Autodesk Inventor part; units mm, degrees
ref_plane "Work Plane2" through (0, 12.5, 0) normal (0, 1, 0) x (1, 0, 0)
ref_plane "YZ Plane" through (0, 0, 0) normal (1, 0, 0) x (0, 1, 0)
ref_plane "XZ Plane" through (0, 0, 0) normal (0, 1, 0) x (-1, 0, 0)
sketch "Sketch1" plane through (0, 0, 0) normal (0, 1, 0) x (-1, 0, 0)
  line L0 (-38.3993, -26.9176) -> (-33.0009, -96.7091)
  line L1 (-33.0009, -96.7091) -> (-8.0012, -96.5869)
  circle A0 centre (-23.2715, -84.2034) radius 5
  circle A1 centre (-27.3538, -47.8392) radius 5
  line L2 (-38.3993, -26.9176) -> (16.6007, -26.9176) construction
  arc A2 (22.7463, 28.593) -> (19.9992, 36.438) centre (15.3555, 30.4084) ccw
  line L3 (-8.0012, -96.5869) -> (22.7463, 28.593)
  line L4 (11.975, 39.0871) -> (13.9695, 41.0816)
  line L5 (13.9695, 41.0816) -> (19.9992, 36.438)
  line L6 (13.9695, 41.0816) -> (16.437, 44.2856)
  line L7 (16.437, 44.2856) -> (13.9695, 41.0816)
  line L8 (13.9695, 41.0816) -> (10.2037, 42.2949)
  line L9 (10.2037, 42.2949) -> (11.1441, 37.4129)
  line L10 (10.3086, 36.328) -> (6.5427, 37.5413)
  line L11 (6.5427, 37.5413) -> (7.4831, 32.6592)
  line L12 (6.6476, 31.5743) -> (2.8817, 32.7876)
  line L13 (2.8817, 32.7876) -> (3.8221, 27.9055)
  line L14 (2.9866, 26.8207) -> (-0.7792, 28.034)
  line L15 (-0.7792, 28.034) -> (0.1612, 23.1519)
  line L16 (-0.6744, 22.067) -> (-4.4402, 23.2803)
  line L17 (-4.4402, 23.2803) -> (-3.4998, 18.3982)
  line L18 (-4.3353, 17.3133) -> (-8.1012, 18.5266)
  line L19 (-8.1012, 18.5266) -> (-7.1608, 13.6446)
  line L20 (-7.9963, 12.5597) -> (-11.7622, 13.773)
  line L21 (-11.7622, 13.773) -> (-10.8218, 8.8909)
  line L22 (-11.6573, 7.806) -> (-15.4231, 9.0193)
  line L23 (-15.4231, 9.0193) -> (-14.4827, 4.1373)
  line L24 (-15.3183, 3.0524) -> (-19.0841, 4.2657)
  line L25 (-19.0841, 4.2657) -> (-18.1437, -0.6164)
  line L26 (10.3086, 36.328) -> (11.1441, 37.4129)
  line L27 (6.6476, 31.5743) -> (7.4831, 32.6592)
  line L28 (2.9866, 26.8207) -> (3.8221, 27.9055)
  line L29 (-0.6744, 22.067) -> (0.1612, 23.1519)
  line L30 (-4.3353, 17.3133) -> (-3.4998, 18.3982)
  line L31 (-7.9963, 12.5597) -> (-7.1608, 13.6446)
  line L32 (-11.6573, 7.806) -> (-10.8218, 8.8909)
  line L33 (-38.3993, -26.9176) -> (-18.1437, -0.6164)
  line L34 (-15.3183, 3.0524) -> (-14.4827, 4.1373)
  point P0 (0, 0)
  dimension "d33" = 10
  dimension "d34" = 10
  dimension "d39" = 6
  dimension "d49" = 70
  dimension "d50" = 25
extrude "Extrusion3" add sketch "Sketch1" along normal blind 25
ref_plane "Work Plane2" through (0, 12.5, 0) normal (0, 1, 0) x (1, 0, 0)
sketch "Sketch4" plane through (0, 12.5, 0) normal (0, 1, 0) x (1, 0, 0)
  line L0 (41.2703, 100.0732) -> (11.3509, 100.0732)
  line L1 (11.3509, 100.0732) -> (11.3509, 24.6286)
  line L2 (11.3509, 24.6286) -> (41.2703, 17.4466)
  line L3 (41.2703, 17.4466) -> (41.2703, 100.0732)
  point P0 (0, 0)
extrude "Extrusion4" cut sketch "Sketch4" along normal mid plane 10
fillet "Fillet5" radius 10 4 edges at (33.0009, 21.25, -96.7091) (33.0009, 3.75, -96.7091) (8.0012, 12.5, -96.5869) (11.3509, 12.5, -24.6286)
properties part number "capit"
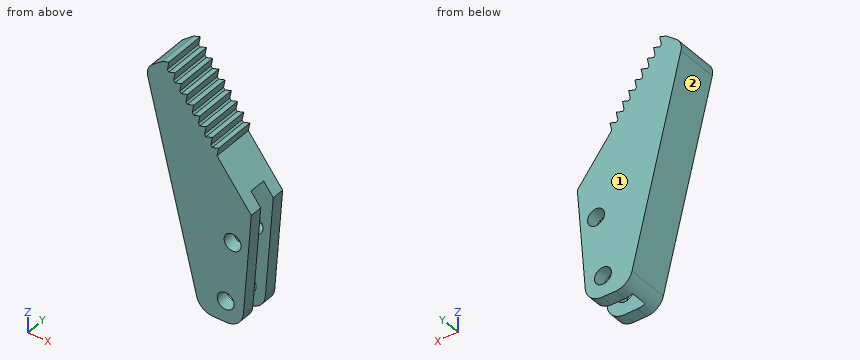
The listing builds one solid part. Answer for the finished solid, in the listing's coordinates (mm). Face numbers are marked on the shaded views. Give positions to 0.01 mm unless a question says otherwise; leave off trailing zeros. Write each loop counter-clockwise with the first axis right and the second up, starting at its lowest first coordinate (ties: lowest second). Pieces come first, ordered by that corner, then holes.
Item 1: Section D-D, the plane y = 22 is taken. Count the separate pieces of the cut face and the enclosed holes in it, plus the area to 3 significant figures.
Item 2: Section B-B, the plane z = -30 is taken. Write down the section's boundary in (x, y), plus the area to 3 significant figures.
Item 3: Section A-A, the plane x = 30 is taken. Write down the section's boundary in (y, z), plus the area to 3 significant figures.
Item 4: Flat-ended cylindrical pins translate along their axes: P1, Ø10, axis at y = 16.5, z = -11.5, coming from the +X side; P2, Ø5, axis at y = 21, z = -45, coming from the -X side; P3, Ø11, axis at y = 11, z = -50.5, coming from the +X side. Find the tip coordinate at first contact, or state that the pin passes through.
Item 5: Find the intervals of material crossed by line 1 along Y through (x, z) = (19, -87.5); line 2 along X through (y, z) = (6.75, -50.5); line 3 along Z through (x, y) = (20, 20.25), in increasing order.
Item 6: Determine the mould class of the marked faces 1 and 2 for opening direction Z: released by +Z, released by -Z, zero draft, split by the parting line, or undercut.
Completed:
1. separate pieces: 1
1. enclosed holes: 2
1. area: 4,390 mm2
2. outline: (-8.35, 0) - (38.16, 0) - (38.16, 7.5) - (11.67, 7.5) - (11.67, 17.5) - (38.16, 17.5) - (38.16, 25) - (-8.35, 25) - close
2. area: 898 mm2
3. outline: (0, -94.47) - (7.5, -94.47) - (7.5, -52.08) - (0, -52.08) - close; (0, -43.6) - (7.5, -43.6) - (7.5, -20.15) - (17.5, -20.15) - (17.5, -43.6) - (25, -43.6) - (25, -16.01) - (0, -16.01) - close; (17.5, -94.47) - (25, -94.47) - (25, -52.08) - (17.5, -52.08) - close
3. area: 1,090 mm2
4. P1: stops at x = 30.38
4. P2: stops at x = -5.28
4. P3: stops at x = 36.9
5. line 1: y = 0 to 7.5, 17.5 to 25
5. line 2: x = -3.32 to 23.12, 31.59 to 36.58
5. line 3: z = -96.65 to -87.98, -80.42 to -3.03
6. face 1: zero draft
6. face 2: released by -Z
